Geometry check sheet. Reference: the model listing, model coordinates, mm. Coordinates: 2 decimals unless noted, no trailing zeros. Order: outer loops, then holes, each group sorted by start corner. A loop starts at its lowest first (then second) coordinate and runs counter-clockwise, first axis right, second up. Notation, with made-up numbers: (65.5, 33) - (106.5, 33) arc R8 cw to (106.5, 40) - close; hole circle Ø10 at (-34, -20.75). An arc over 180 degrees is marked (long way). Return JSON: item names as keys, results as strings. Group by question number.
Item 1: Scan lines: probe 1 along Y at (x, z) = (55, 3.65); probe 2 along X at (y, z) = (-1.5, 3.25); probe 3 along X at (y, z) = (2, -0.25). Record each from-to range of solid material in increasing order.
Item 2: Section check D-D on y = -1.75. Enter the section's corners in (x, z), then the cut area to 3 significant figures.
Item 3: Section check C-C on z = -2. Enter the section's corners in (x, y), then the cut area to 3 significant figures.
Item 4: Gauge pin test, flat end, axial feed: pin 1 (12 mm diameter, centred on x = 1, y = 1.5, fed in from -Z). Record the tip position at first contact, or that the pin passes through.
Item 5: Section check A-A on y = -7.75. Enter the section's corners in (x, z), then the cut area to 3 significant figures.
Item 6: Section check B-B on x = -55. Enter the section's corners in (y, z), then the cut area to 3 significant figures.
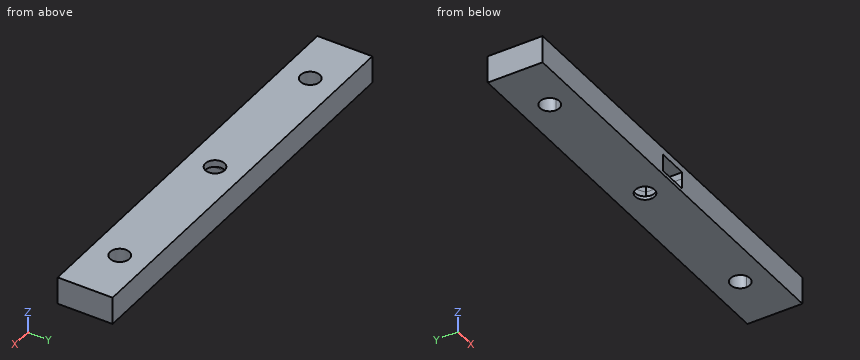
from build123d import *

# Parameters (mm, degrees)
F0_W          = 11.124
F0_H          = 6.4224443945
F1_DEPTH      = 5
F1_DEPTH_BACK = 5
F2_D          = 7
F2_DEPTH      = 5.001
F3_D          = 7
F4_DEPTH      = 2.5
F4_DEPTH_BACK = 3.7


with BuildPart() as f1:
    # F0 (on Top) → F1 (new body, two sides)
    with BuildSketch(Plane.XY) as f1_sk:
        Polygon((-5.562, 10), (-75, 10), (-75, -10), (-5.562, -10), (-5.562, -3.2112221972), (-5.562, 3.2112221972), align=None)
        Polygon((75, 10), (5.562, 10), (5.562, 3.2112221972), (5.562, -3.2112221972), (5.562, -10), (75, -10), align=None)
        Polygon((0, 6.4224443945), (-5.562, 3.2112221972), (5.562, 3.2112221972), align=None)
        Polygon((5.562, 10), (-5.562, 10), (-5.562, 3.2112221972), (0, 6.4224443945), (5.562, 3.2112221972), align=None)
        Polygon((-5.562, -3.2112221972), (-5.562, -10), (5.562, -10), (5.562, -3.2112221972), (0, -6.4224443945), align=None)
        Polygon((5.562, -3.2112221972), (-5.562, -3.2112221972), (0, -6.4224443945), align=None)
        Rectangle(F0_W, F0_H)
    extrude(amount=F1_DEPTH)
    extrude(f1_sk.sketch, amount=-F1_DEPTH_BACK)

    # F2 (through all, one way)
    with BuildSketch(Plane.XY):
        with Locations((-55, 0), (55, 0), (0, 0)):
            Circle(F2_D / 2)
    extrude(amount=-F2_DEPTH, mode=Mode.SUBTRACT)

    # F3 (through all)
    with Locations(Plane(origin=(0, 0, 0), x_dir=(1, 0, 0), z_dir=(0, 0, -1))):
        with Locations((55, 0), (-55, 0), (0, 0)):
            Hole(F3_D / 2)

    # F0 (on Top) → F4 (cut, two sides)
    with BuildSketch(Plane.XY) as f4_sk:
        Polygon((0, 6.4224443945), (-5.562, 3.2112221972), (5.562, 3.2112221972), align=None)
        Rectangle(F0_W, F0_H)
        Polygon((5.562, -3.2112221972), (-5.562, -3.2112221972), (0, -6.4224443945), align=None)
        Polygon((-5.562, -3.2112221972), (-5.562, -10), (5.562, -10), (5.562, -3.2112221972), (0, -6.4224443945), align=None)
    extrude(amount=F4_DEPTH, mode=Mode.SUBTRACT)
    extrude(f4_sk.sketch, amount=-F4_DEPTH_BACK, mode=Mode.SUBTRACT)


solid = f1.part
Computed:
{
 "1": {"probe 1": "y = -10 to -3.5, 3.5 to 10", "probe 2": "x = -75 to -58.16, -51.84 to -3.16, 3.16 to 51.84, 58.16 to 75", "probe 3": "x = -75 to -57.87, -52.13 to -5.56, 5.56 to 52.13, 57.87 to 75"},
 "2": {"outline": "(-75, -5) - (-58.03, -5) - (-58.03, 5) - (-75, 5) - close; (-51.97, -5) - (-3.03, -5) - (-3.03, -3.7) - (-5.56, -3.7) - (-5.56, 2.5) - (-3.03, 2.5) - (-3.03, 5) - (-51.97, 5) - close; (3.03, -5) - (51.97, -5) - (51.97, 5) - (3.03, 5) - (3.03, 2.5) - (5.56, 2.5) - (5.56, -3.7) - (3.03, -3.7) - close; (58.03, -5) - (75, -5) - (75, 5) - (58.03, 5) - close", "area": "1,290 mm²"},
 "3": {"outline": "(-75, -10) - (-5.56, -10) - (-5.56, 3.21) - (0, 6.42) - (5.56, 3.21) - (5.56, -10) - (75, -10) - (75, 10) - (-75, 10) - close; hole circle Ø7 at (-55, 0); hole circle Ø7 at (55, 0)", "area": "2,760 mm²"},
 "4": {"pin 1": "stops at z = -5"},
 "5": {"outline": "(-75, -5) - (75, -5) - (75, 5) - (-75, 5) - close; hole (-5.56, -3.7) - (5.56, -3.7) - (5.56, 2.5) - (-5.56, 2.5) - close", "area": "1,430 mm²"},
 "6": {"outline": "(-10, -5) - (-3.5, -5) - (-3.5, 5) - (-10, 5) - close; (3.5, -5) - (10, -5) - (10, 5) - (3.5, 5) - close", "area": "130 mm²"}
}
